The model under review builds one solid part; all positions refer to its coordinate system, in mm. Coordinates: 2 decimals unless noted, no trailing zeros. Loops run counter-clockwise (first coordinate to the right, second up) from the corner with the lowest first, then second, coordinate; pieces in that order, holes last. Notation, with made-up numbers: M -35,35.5 L -3,35.5 A24 ccw -3,46.5 Z; hole C 30,35.25 d2. An arc over 180 degrees is marked long. Write item = value, one per line. Start each with the question number.
Q1. We need section C-C on y = 84. Give the boundary of the cut face in (x, z), and give its area (3 significant figures).
Q2. Wall thickness on probe 1 along Z at (x, y) = (3.55, 103.5); probe 2 along Z at (x, y) = (3.2, 47): over which ranges is each line inside the solid? List them lowest first.
Q3. Clearance check with flat-ended pins moving along their axes: pin 1 Ø0.9 at (x, y) = (4, 127.5) entering from +Z; pin 2 Ø1.2 at (x, z) = (3.5, -37) entering from +Y; pin 3 Ø1.5 at (x, z) = (5, -9) entering from +Y. State where each tip first meets the part, or that it passes through.
Q4. We need section B-B on x = 5.5. Give the boundary of the cut face in (y, z), and give its area (3 significant figures).
Q5. We need section A-A on y = 49.5. Give the boundary of the cut face in (x, z).
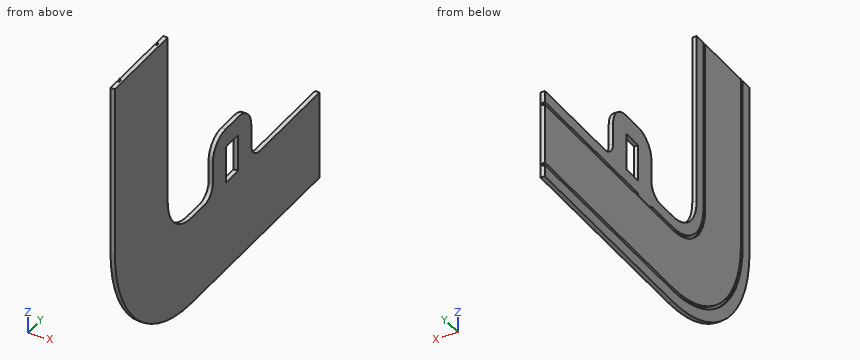
from build123d import *

# Parameters (mm, degrees)
BOSS_EXTRUDE1_DEPTH = 3
CUT_EXTRUDE1_DEPTH  = 1.5
SKETCH5_W           = 40
SKETCH5_H           = 45
BOSS_EXTRUDE2_DEPTH = 3
SKETCH6_W           = 26
SKETCH6_H           = 14
CUT_EXTRUDE2_DEPTH  = 3
FILLET1_R           = 15
SKETCH7_W           = 10.438197785
SKETCH7_H           = 15.5
SKETCH7_W_2         = 18.220797936
BOSS_EXTRUDE3_DEPTH = 3
FILLET2_R           = 10


with BuildPart() as part:
    # Sketch1 → Boss-Extrude1 (new body)
    with BuildSketch(Plane(origin=(0, 0, 0), x_dir=(0, 0, -1), z_dir=(1, 0, 0))):
        with BuildLine():
            Line((0, -28), (-120, -28))
            Line((-120, -28), (-120, -90))
            Line((-120, -90), (0, -90))
            ThreePointArc((0, -90), (63.639610307, -63.639610307), (90, 0))
            Line((90, 0), (90, 150))
            Line((90, 150), (28, 150))
            Line((28, 150), (28, 0))
            ThreePointArc((28, 0), (19.798989873, -19.798989873), (0, -28))
        make_face()
    extrude(amount=BOSS_EXTRUDE1_DEPTH)

    # Sketch2 → Cut-Extrude1 (cut)
    with BuildSketch(Plane(origin=(3, 0, 0), x_dir=(0, 0, -1), z_dir=(1, 0, 0))):
        with BuildLine():
            Line((0, -38), (-120, -38))
            Line((-120, -38), (-120, -36))
            Line((-120, -36), (0, -36))
            ThreePointArc((0, -36), (25.455844123, -25.455844123), (36, 0))
            Line((36, 0), (36, 150))
            Line((36, 150), (38, 150))
            Line((38, 150), (38, 0))
            ThreePointArc((38, 0), (26.870057685, -26.870057685), (0, -38))
        make_face()
        with BuildLine():
            Line((0, -80), (-120, -80))
            Line((-120, -80), (-120, -82))
            Line((-120, -82), (0, -82))
            ThreePointArc((0, -82), (57.982756057, -57.982756057), (82, 0))
            Line((82, 0), (82, 150))
            Line((82, 150), (80, 150))
            Line((80, 150), (80, 0))
            ThreePointArc((80, 0), (56.568542495, -56.568542495), (0, -80))
        make_face()
    extrude(amount=-CUT_EXTRUDE1_DEPTH, mode=Mode.SUBTRACT)


with BuildPart() as body_2:
    # Mirror1: mirrored copy
    add(part.part.mirror(Plane(origin=(3, 0, 0), x_dir=(0, 0, 1), z_dir=(1, 0, 0))))



with BuildPart() as body_2_2:
    # Sketch5 → Boss-Extrude2 (new body)
    with BuildSketch(Plane(origin=(6, 0, 0), x_dir=(0, 0, -1), z_dir=(1, 0, 0))):
        with Locations((8, 47.5)):
            Rectangle(SKETCH5_W, SKETCH5_H)
    extrude(amount=-BOSS_EXTRUDE2_DEPTH)

    # Sketch6 → Cut-Extrude2 (cut)
    with BuildSketch(Plane(origin=(6, 0, 0), x_dir=(0, 0, -1), z_dir=(1, 0, 0))):
        with Locations((14, 47.5)):
            Rectangle(SKETCH6_W, SKETCH6_H)
    extrude(amount=-CUT_EXTRUDE2_DEPTH, mode=Mode.SUBTRACT)

    # Fillet1
    fillet1_edges = [body_2_2.edges().sort_by_distance(p)[0] for p in [
        (4.5, 25, 12),
        (4.5, 70, 12),
    ]]
    fillet(fillet1_edges, radius=FILLET1_R)


with BuildPart() as body_2_1:
    add(body_2.part)

    add(body_2_2.part)  # Boss-Extrude3 merges body 2 2
    # Sketch7 → Boss-Extrude3 (add)
    with BuildSketch(Plane(origin=(6, 0, 0), x_dir=(0, 0, -1), z_dir=(1, 0, 0))):
        with Locations((26.467997442, 62.25)):
            Rectangle(SKETCH7_W, SKETCH7_H)
        with Locations((28.397040912, 32.75)):
            Rectangle(SKETCH7_W_2, SKETCH7_H)
    extrude(amount=-BOSS_EXTRUDE3_DEPTH)

    # Fillet2
    fillet2_edges = [body_2_1.edges().sort_by_distance(p)[0] for p in [
        (4.5, 70, -28),
        (4.5, 25, -28),
    ]]
    fillet(fillet2_edges, radius=FILLET2_R)


solid = body_2_1.part
Returned:
q1.outline = M 3,-90 L 6,-90 L 6,-28 L 3,-28 L 3,-36 L 4.5,-36 L 4.5,-38 L 3,-38 L 3,-80 L 4.5,-80 L 4.5,-82 L 3,-82 Z
q1.area = 180 mm^2
q2.probe_1 = -90 to -82, -80 to -38, -36 to -28
q2.probe_2 = -90 to -82, -80 to -38, -36 to -27, -1 to 12
q3.pin_1 = -28
q3.pin_2 = 40.5
q3.pin_3 = 70
q4.outline = M -90,0 A90 ccw 0,-90 L 150,-90 L 150,-28 L 80,-28 A10 cw 70,-18 L 70,-3 A15 ccw 55,12 L 40,12 A15 ccw 25,-3 L 25,-18 A10 cw 15,-28 L 0,-28 A28 cw -28,0 L -28,120 L -90,120 Z; hole M 40.5,-27 L 54.5,-27 L 54.5,-1 L 40.5,-1 Z
q4.area = 23,900 mm^2
q5.outline = M 3,-90 L 6,-90 L 6,-27 L 3,-27 L 3,-36 L 4.5,-36 L 4.5,-38 L 3,-38 L 3,-80 L 4.5,-80 L 4.5,-82 L 3,-82 Z; M 3,-1 L 6,-1 L 6,12 L 3,12 Z
